Could you check a few things on this model? Use its own coordinates, in mm. Face numbers are marked on the shaded views. A direction names the side the tool comes from. Give positions to 0.01 mm unless a question says otherwise; leave off trailing zeros. Loops run counter-clockwise (first coordinate to the right, second up) from the corner with the lowest first, then second, coordinate; pieces in that order, holes last. Notation, with made-up numbers: (17.25, 80.5) - (37.25, 80.5) arc R10 ccw to (37.25, 95.5) - close; hole circle Ø9 at (38, 81). An arc over 180 degrees is marked (long way). One line per item, written item: value. Start each with the question number.
Q1. I want a section at A-A (y = 27). Please give me the cut outline in (x, z), then the cut area to 3 significant figures.
Q2. I'm going to push flat-ended pins straight in: P1, Ø1, axis at y = 5, z = 11.5, coming from the +X side; P2, Ø5.5, axis at x = 61, y = 33, coming from the +Z side; P3, Ø11, axis at x = 123.77, z = 0, coming from the +Y side. Where does each tip first touch, or does it pass through?
Q3. I want a section at B-B (z = 0). Count the separate pieces of the cut face and the enclosed holes in it, then the cut area to 3 significant figures.
Q4. If we mould it in two halves opening along X, with no side actions, what happens to the marked faces 4, 5 and 6? For each: released by +X, released by -X, zero draft, split by the parting line, or undercut.
Q5. For the marked faces 1, 2 and 3, which set-ups out of +Z, -Z, +X, -X, +Y, -Y let a thin tool reach every point of the face, with its end or its side?
Q6. If I drill on line 1 (X direction, y = 3.75, z = 0); line 2 (X direction, y = 23, z = 0); line 3 (X direction, y = 5, z = 32), over which ranges is the centre line in solid material (lowest first)? Write a range as from..to.
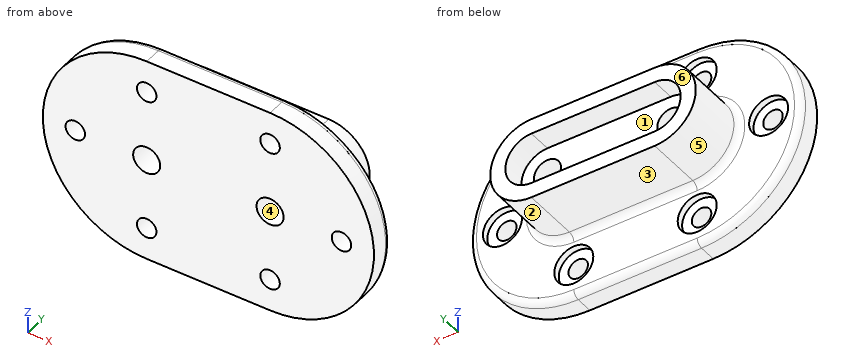
```python
from build123d import *

# Parameters (mm, degrees)
EXTRUDE_1_DEPTH     = 11
SKETCH_4_R          = 9
SKETCH_4_R_2        = 4.5
CUT_EXTRUDE_1_DEPTH = 3
SKETCH_4_3_R        = 4.5
CUT_EXTRUDE_2_DEPTH = 11
EXTRUDE_3_DEPTH     = 40
EXTRUDE_4_DEPTH     = 29
SKETCH_8_R          = 6.25
CUT_EXTRUDE_3_DEPTH = 150.66913845
FILLET_1_R          = 3
FILLET_2_R          = 3


with BuildPart() as part:
    # Sketch 1 → Extrude 1 (new body)
    with BuildSketch(Plane(origin=(0, 0, 0), x_dir=(1, 0, 0), z_dir=(0, 1, 0))):
        with BuildLine():
            Line((33.765453209, 48), (90.765453209, 48))
            ThreePointArc((90.765453209, 48), (138.765453209, 0), (90.765453209, -48))
            Line((90.765453209, -48), (33.765453209, -48))
            ThreePointArc((33.765453209, -48), (-14.234546791, 0), (33.765453209, 48))
        make_face()
    extrude(amount=EXTRUDE_1_DEPTH)

    # Sketch 4 → Cut-Extrude 1 (cut)
    # profile 1 of 6: a face of its own
    with BuildSketch(Plane(origin=(0, 11, 0), x_dir=(1, 0, 0), z_dir=(0, 1, 0))):
        with Locations(Location((0.765453209, 0, 0), (0, 0, 270))):
            Circle(SKETCH_4_R)
        with Locations(Location((0.765453209, 0, 0), (0, 0, 270))):
            Circle(SKETCH_4_R_2, mode=Mode.SUBTRACT)
    # profile 2 of 6: a face of its own
    with BuildSketch(Plane(origin=(0, 11, 0), x_dir=(1, 0, 0), z_dir=(0, 1, 0))):
        with Locations(Location((33.765453209, 33, 0), (0, 0, 270))):
            Circle(SKETCH_4_R)
        with Locations(Location((33.765453209, 33, 0), (0, 0, 270))):
            Circle(SKETCH_4_R_2, mode=Mode.SUBTRACT)
    # profile 3 of 6: a face of its own
    with BuildSketch(Plane(origin=(0, 11, 0), x_dir=(1, 0, 0), z_dir=(0, 1, 0))):
        with Locations(Location((90.765453209, 33, 0), (0, 0, 270))):
            Circle(SKETCH_4_R)
        with Locations(Location((90.765453209, 33, 0), (0, 0, 270))):
            Circle(SKETCH_4_R_2, mode=Mode.SUBTRACT)
    # profile 4 of 6: a face of its own
    with BuildSketch(Plane(origin=(0, 11, 0), x_dir=(1, 0, 0), z_dir=(0, 1, 0))):
        with Locations(Location((123.765453209, 0, 0), (0, 0, 270))):
            Circle(SKETCH_4_R)
        with Locations(Location((123.765453209, 0, 0), (0, 0, 270))):
            Circle(SKETCH_4_R_2, mode=Mode.SUBTRACT)
    # profile 5 of 6: a face of its own
    with BuildSketch(Plane(origin=(0, 11, 0), x_dir=(1, 0, 0), z_dir=(0, 1, 0))):
        with Locations(Location((90.765453209, -33, 0), (0, 0, 270))):
            Circle(SKETCH_4_R)
        with Locations(Location((90.765453209, -33, 0), (0, 0, 270))):
            Circle(SKETCH_4_R_2, mode=Mode.SUBTRACT)
    # profile 6 of 6: a face of its own
    with BuildSketch(Plane(origin=(0, 11, 0), x_dir=(1, 0, 0), z_dir=(0, 1, 0))):
        with Locations(Location((33.765453209, -33, 0), (0, 0, 270))):
            Circle(SKETCH_4_R)
        with Locations(Location((33.765453209, -33, 0), (0, 0, 270))):
            Circle(SKETCH_4_R_2, mode=Mode.SUBTRACT)
    extrude(amount=-CUT_EXTRUDE_1_DEPTH, mode=Mode.SUBTRACT)

    # Sketch 4_3 → Cut-Extrude 2 (cut)
    with BuildSketch(Plane(origin=(0, 11, 0), x_dir=(1, 0, 0), z_dir=(0, 1, 0))):
        with Locations(Location((33.765453209, -33, 0), (0, 0, 270))):
            Circle(SKETCH_4_3_R)
        with Locations(Location((0.765453209, 0, 0), (0, 0, 270))):
            Circle(SKETCH_4_3_R)
        with Locations(Location((33.765453209, 33, 0), (0, 0, 270))):
            Circle(SKETCH_4_3_R)
        with Locations(Location((90.765453209, 33, 0), (0, 0, 270))):
            Circle(SKETCH_4_3_R)
        with Locations(Location((123.765453209, 0, 0), (0, 0, 270))):
            Circle(SKETCH_4_3_R)
        with Locations(Location((90.765453209, -33, 0), (0, 0, 270))):
            Circle(SKETCH_4_3_R)
    extrude(amount=-CUT_EXTRUDE_2_DEPTH, mode=Mode.SUBTRACT)

    # Sketch 1_5 → Extrude 3 (add)
    with BuildSketch(Plane(origin=(0, 0, 0), x_dir=(1, 0, 0), z_dir=(0, 1, 0))):
        with BuildLine():
            Line((33.765453209, -19), (90.765453209, -19))
            ThreePointArc((90.765453209, -19), (109.765453209, 0), (90.765453209, 19))
            Line((90.765453209, 19), (33.765453209, 19))
            ThreePointArc((33.765453209, 19), (14.765453209, 0), (33.765453209, -19))
        make_face()
        with BuildLine():
            ThreePointArc((90.765453209, -12), (102.765453209, 0), (90.765453209, 12))
            Line((90.765453209, 12), (33.765453209, 12))
            ThreePointArc((33.765453209, 12), (21.765453209, 0), (33.765453209, -12))
            Line((33.765453209, -12), (90.765453209, -12))
        make_face(mode=Mode.SUBTRACT)
    extrude(amount=EXTRUDE_3_DEPTH)

    # Sketch 1_6 → Extrude 4 (add)
    with BuildSketch(Plane(origin=(0, 0, 0), x_dir=(1, 0, 0), z_dir=(0, 1, 0))):
        with BuildLine():
            Line((33.765453209, -12), (90.765453209, -12))
            ThreePointArc((90.765453209, -12), (102.765453209, 0), (90.765453209, 12))
            Line((90.765453209, 12), (33.765453209, 12))
            ThreePointArc((33.765453209, 12), (21.765453209, 0), (33.765453209, -12))
        make_face()
    extrude(amount=EXTRUDE_4_DEPTH)

    # Sketch 8 → Cut-Extrude 3 (cut, through all)
    with BuildSketch(Plane(origin=(0, 29, 0), x_dir=(1, 0, 0), z_dir=(0, 1, 0))):
        with Locations(Location((33.765453209, 0, 0), (0, 0, 270))):
            Circle(SKETCH_8_R)
        with Locations(Location((90.765453209, 0, 0), (0, 0, 270))):
            Circle(SKETCH_8_R)
    extrude(amount=-CUT_EXTRUDE_3_DEPTH, mode=Mode.SUBTRACT)

    # Fillet 1
    fillet_1_edges = [part.edges().sort_by_distance(p)[0] for p in [
        (138.765453209, 11, 0),
        (62.265453209, 11, -48),
        (-14.234546791, 11, 0),
        (62.265453209, 11, 48),
    ]]
    fillet(fillet_1_edges, radius=FILLET_1_R)

    # Fillet 2
    fillet_2_edges = [part.edges().sort_by_distance(p)[0] for p in [
        (62.265453209, 11, 19),
        (109.765453209, 11, 0),
        (14.765453209, 11, 0),
        (62.265453209, 11, -19),
    ]]
    fillet(fillet_2_edges, radius=FILLET_2_R)


solid = part.part
```
Worked answers:
1. outline: (33.77, -19) - (90.77, -19) arc R19 ccw to (90.77, 19) - (33.77, 19) arc R19 ccw to start; hole circle Ø12.5 at (33.77, 0); hole circle Ø12.5 at (90.77, 0)
1. area: 3,050 mm²
2. P1: stops at x = 137.49
2. P2: stops at z = 19
2. P3: stops at y = 8
3. separate pieces: 5
3. enclosed holes: 0
3. area: 2,570 mm²
4. face 4: undercut
4. face 5: released by -X
4. face 6: zero draft
5. face 1: +Y
5. face 2: +X, +Y
5. face 3: -Z, +X, -X, +Y
6. line 1: x = -14.23..-3.73, 5.27..27.52, 40.02..84.52, 97.02..119.27, 128.27..138.77
6. line 2: x = 14.77..27.52, 40.02..84.52, 97.02..109.77
6. line 3: x = -2.01..29.38, 38.15..86.38, 95.15..126.54
